Model file for the job. Use its own axes, mm. Face numbers are marked on the shaded views. Coordinates: 2 decimals unless noted, no trailing zeros. Order: outer loops, then holes, each group sorted by start corner. A loop starts at its lowest first (then second) coordinate and runs counter-clockwise, first axis right, second up. Notation, with made-up numbers: (29.5, 57.25) -> (61.5, 57.25) arc R15 ccw to (61.5, 83.25) -> close; hole circle Ø2 at (40, 23.5). An arc over 180 degrees is marked (long way). Write item = value, one per line. Start each with the question number.
Q1. Wall check: line 1 (Z direction, x = -3.5, y = 5.75); line 2 (Z direction, x = 3.5, y = -1); line 3 (X direction, y = -2.75, z = 4.75). Give the ranges that are in metal, low to high. Write a range as from..to.
Q2. Mould opens along Z. For the marked faces 1, 2, 3 and 4 say: +Z half, -Z half, draft (parallel to the pull), parting line (faces both ways), or undercut.
Q3. Cut at C-C, the plane z = 9.5. List the corners of the cut face in (x, y), plus the area to 3 significant figures.
Q4. Flat gauge pins, fed straight in: pin 1 (5 mm diameter, centred on x = 3, z = 9.5, fed in from +Y); pin 2 (5 mm diameter, centred on y = 1.5, z = 10.5, fed in from -X); pin 3 (6 mm diameter, centred on y = 4.5, z = 6, fed in from -X). Where does each tip first touch, or does it go through?
from build123d import *

# Parameters (mm, degrees)
SKETCH1_R      = 8.89
EXTRUDE1_DEPTH = 1.524
SKETCH2_R      = 1.9558
EXTRUDE2_DEPTH = 3.175
SKETCH3_R      = 3.81
EXTRUDE3_DEPTH = 7.9375
SKETCH4_R      = 2.54
EXTRUDE4_DEPTH = 3.175
FILLET1_R      = 2.54
CHAMFER4_SIZE  = 1.27
FILLET2_R      = 1.524


with BuildPart() as part:
    # Sketch1 → Extrude1 (new body)
    with BuildSketch(Plane.XY):
        Circle(SKETCH1_R)
    extrude(amount=EXTRUDE1_DEPTH)

    # Sketch2 → Extrude2 (add)
    with BuildSketch(Plane.XY.offset(1.524)):
        Circle(SKETCH2_R)
    extrude(amount=EXTRUDE2_DEPTH)

    # Sketch3 → Extrude3 (add)
    with BuildSketch(Plane.XY.offset(4.699)):
        Circle(SKETCH3_R)
    extrude(amount=EXTRUDE3_DEPTH)

    # Sketch4 → Extrude4 (add)
    with BuildSketch(Plane.XY.offset(12.6365)):
        with Locations(Location((0, 0, 0), (0, 0, 180))):
            Circle(SKETCH4_R)
    extrude(amount=EXTRUDE4_DEPTH)

    # Fillet1
    fillet1_edges = [part.edges().sort_by_distance(p)[0] for p in [
        (2.54, 0, 15.8115),
    ]]
    fillet(fillet1_edges, radius=FILLET1_R)

    # Chamfer4
    chamfer4_edges = [part.edges().sort_by_distance(p)[0] for p in [
        (-3.81, 0, 12.6365),
    ]]
    chamfer(chamfer4_edges, length=CHAMFER4_SIZE - 0.0001)  # a hair under: the kernel refuses the full size

    # Fillet2
    fillet2_edges = [part.edges().sort_by_distance(p)[0] for p in [
        (-8.89, 0, 0),
    ]]
    fillet(fillet2_edges, radius=FILLET2_R - 0.0001)  # a hair under: the kernel refuses the full size


solid = part.part
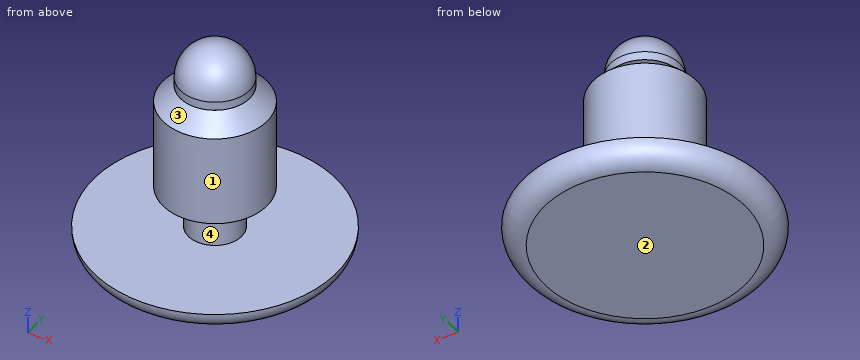
Here are the results:
q1.line_1 = 0..1.52
q1.line_2 = 0..1.52, 4.7..11.54
q1.line_3 = -2.64..2.64
q2.face_1 = draft
q2.face_2 = -Z half
q2.face_3 = +Z half
q2.face_4 = undercut
q3.outline = circle Ø7.62 at (0, 0)
q3.area = 45.6 mm²
q4.pin_1 = 3.78
q4.pin_2 = -3.81
q4.pin_3 = -3.5
